```python
from build123d import *

# Parameters (mm, degrees)
F1_DEPTH = 38.1
F6_DEPTH = 38.1
F7_DEPTH = 38.1
F8_W     = 25.4
F8_H     = 7.62
F9_DEPTH = 38.1


with BuildPart() as f1:
    # F0 (on Front) → F1 (new body)
    with BuildSketch(Plane.XZ):
        Polygon((6.35, 38.1), (0, 0), (6.35, 0), (11.43, 22.225), (16.51, 9.525), (21.59, 9.525), (26.67, 22.225), (31.75, 0), (38.1, 0), (31.75, 38.1), (25.4, 38.1), (19.05, 22.225), (12.7, 38.1), align=None)
        Polygon((0, 38.1), (0, 0), (6.35, 38.1), align=None)
        Polygon((11.43, 22.225), (6.35, 0), (31.75, 0), (26.67, 22.225), (21.59, 9.525), (16.51, 9.525), align=None)
        Polygon((25.4, 38.1), (12.7, 38.1), (19.05, 22.225), align=None)
        Polygon((31.75, 38.1), (38.1, 0), (38.1, 38.1), align=None)
    extrude(amount=-F1_DEPTH)

    # F5 (on offset) → F6 (cut)
    with BuildSketch(Plane.YZ.offset(38.1)):
        Polygon((31.75, 38.1), (6.35, 38.1), (11.43, 13.704411), (16.51, 28.575), (21.59, 28.575), (26.67, 14.422566), align=None)
        Polygon((0, 38.1), (0, 0), (6.35, 0), align=None)
        Polygon((19.05, 15.875), (12.7, 0), (25.4, 0), align=None)
        Polygon((38.1, 0), (38.1, 38.1), (31.75, 0), align=None)
    extrude(amount=-F6_DEPTH, mode=Mode.SUBTRACT)

    # F0 (on Front) → F7 (cut)
    with BuildSketch(Plane.XZ):
        Polygon((0, 38.1), (0, 0), (6.35, 38.1), align=None)
        Polygon((25.4, 38.1), (12.7, 38.1), (19.05, 22.225), align=None)
        Polygon((31.75, 38.1), (38.1, 0), (38.1, 38.1), align=None)
        Polygon((11.43, 22.225), (6.35, 0), (31.75, 0), (26.67, 22.225), (21.59, 9.525), (16.51, 9.525), align=None)
    extrude(amount=-F7_DEPTH, mode=Mode.SUBTRACT)

    # F8 (on offset) → F9 (cut)
    with BuildSketch(Plane.XY.offset(38.1)):
        with Locations((25.4, 26.67)):
            Rectangle(F8_W, F8_H)
        with Locations((12.7, 11.43)):
            Rectangle(F8_W, F8_H)
    extrude(amount=-F9_DEPTH, mode=Mode.SUBTRACT)


solid = f1.part
```
Can you work these out from the model? Positions are in its coordinate system, mm. A direction names the side the tool comes from. Give positions to 0.01 mm unless a question says otherwise; leave off trailing zeros. Loops run counter-clockwise (first coordinate to the right, second up) from the corner with the lowest first, then second, coordinate; pieces in that order, holes last. Notation, with made-up numbers: M -27,68 L 27,68 A32 ccw 27,97 Z; hole C 3.5,-26.5 d9. An arc over 180 degrees is marked long. Use CSV: the item, a comma, the result in double quotes. Start each with the question number.
1. If we mould it in two halves opening along Y, with no side actions, what happens to faces 4 (the face through (8.824, 29.174, 26.096)), 5 (the face through (28.68, 32.38, 13.43))? For each: released by +Y, released by -Y, zero draft, split by the parting line, or undercut.
2. On a 3-axis mill with a long thin cutter (end or side, diameter ignored), from which of +Z, -Z, +X, -X, +Y, -Y can I reach the whole of each face in a straight line? I mean faces 1 (the face through (27.147, 22.216, 26.831)), 2 (the face through (33.2, 15.9, 8)), 3 (the face through (9.49, 25.21, 13.74)). Say none if no direction works.
3. Imagine slicing it at C-C, the plane x = 21. Count the separate pieces of the cut face and the enclosed holes in it, plus the area to 3 significant figures.
4. Imagine slicing it at A-A, the plane z = 7.5. Write out the boundary of the cut face in (x, y).
5. If I drill on L1, parallel to X at y = 4.5, z = 14; L2, parallel to Y at x = 33, z = 20.5; L3, parallel to Y at x = 21, z = 15.5, over which ranges is the centre line in solid material (lowest first)?
6. For P1, Ø4, axis at x = 16.5, y = 13.5, coming from the -Z side (3 decimals); P2, Ø1, axis at x = 13.5, z = 26, coming from the -Y side; P3, Ø7.5, axis at x = 29, z = 17.5, coming from the -Y side, each with a flat end and sliding along its axis, tell me the tip position at first contact or that it passes through.
7. Imagine slicing it at B-B, the plane z = 30. Write out the boundary of the cut face in (x, y).
Response values:
1,face 4,"undercut"
1,face 5,"zero draft"
2,face 1,"+Z, +X, -X"
2,face 2,"-Z, +X, -X"
2,face 3,"-Z, +Y, -Y"
3,separate pieces,"3"
3,enclosed holes,"0"
3,area,"268 mm^2"
4,outline,"M 1.25,5.1 L 8.06,5.1 L 8.06,7.62 L 1.25,7.62 Z; M 1.25,15.24 L 8.06,15.24 L 8.06,15.7 L 1.25,15.7 Z; M 1.25,22.4 L 8.06,22.4 L 8.06,33 L 1.25,33 Z; M 30.04,5.1 L 36.85,5.1 L 36.85,15.7 L 30.04,15.7 Z; M 30.04,22.4 L 36.85,22.4 L 36.85,22.86 L 30.04,22.86 Z; M 30.04,30.48 L 36.85,30.48 L 36.85,33 L 30.04,33 Z"
5,L1,"2.33 to 9.55, 14.72 to 23.38, 28.55 to 35.77"
5,L2,"2.93 to 10.01, 13.75 to 22.86, 30.48 to 35.17"
5,L3,"3.77 to 7.62, 15.24 to 18.9, 19.2 to 22.86, 30.48 to 34.33"
6,P1,"z = 9.525"
6,P2,"y = 1.93"
6,P3,"y = 2.81"
7,outline,"M 5,1.35 L 15.94,1.35 L 15.94,7.62 L 5,7.62 Z; M 5,30.01 L 12.7,30.01 L 12.7,30.48 L 15.94,30.48 L 15.94,36.75 L 5,36.75 Z; M 22.16,1.35 L 33.1,1.35 L 33.1,8.04 L 25.4,8.04 L 25.4,7.62 L 22.16,7.62 Z; M 22.16,30.48 L 33.1,30.48 L 33.1,36.75 L 22.16,36.75 Z"
